Build history of the part. All positions in model axes, mm. Face numbers are marked on the shaded views. A direction names the side the tool comes from. Coordinates: 2 decimals unless noted, no trailing zeros. Write each loop counter-clockwise with the first axis right and the second up, starting at its lowest first coordinate (ties: lowest second). Pieces come first, ordered by that corner, then holes.
Autodesk Inventor part; units mm, degrees
ref_plane "YZ Plane" through (0, 0, 0) normal (1, 0, 0) x (0, 1, 0)
ref_plane "XZ Plane" through (0, 0, 0) normal (0, 1, 0) x (-1, 0, 0)
ref_plane "XY Plane" through (0, 0, 0) normal (0, 0, 1) x (1, 0, 0)
sketch "Sketch1" plane through (0, 0, 0) normal (0, 1, 0) x (-1, 0, 0)
  line L0 (10.6592, 57.15) -> (-7.8828, 57.15)
  line L1 (-7.8828, 57.15) -> (-7.8828, -12.7)
  line L2 (-7.8828, -12.7) -> (10.6592, -12.7)
  line L3 (10.6592, 50.8) -> (-1.5328, 50.8)
  line L4 (-1.5328, 50.8) -> (-1.5328, 25.4)
  line L5 (-1.5328, 25.4) -> (10.6592, 25.4)
  line L6 (10.6592, 19.05) -> (-1.5328, 19.05)
  line L7 (-1.5328, 19.05) -> (-1.5328, -6.35)
  line L8 (-1.5328, -6.35) -> (10.6592, -6.35)
  line L9 (10.6592, -12.7) -> (10.6592, -6.35)
  line L10 (10.6592, 19.05) -> (10.6592, 25.4)
  line L11 (10.6592, 50.8) -> (10.6592, 57.15)
  point P0 (0, 0)
  dimension "d0" = 18.542
  dimension "d3" = 6.35
  dimension "d4" = 6.35
  dimension "d5" = 6.35
  dimension "d7" = 0
  dimension "d8" = 25.4
  dimension "d9" = 25.4
  dimension "d25" = 0
  dimension "d26" = 0
extrude "Extrusion1" add sketch "Sketch1" along normal blind 101.6
sketch "Sketch2" plane through (1.5328, 0, -6.35) normal (-1, 0, 0) x (0, 0, 1)
  line L0 (0, 0) -> (0, 101.6)
  line L1 (0, 0) -> (25.4, 0)
  point P0 (6.35, 0)
  point P1 (12.7, 25.4)
  point P2 (12.7, 50.8)
  point P3 (12.7, 76.2)
  dimension "d12" = 12.7
  dimension "d13" = 25.4
  dimension "d14" = 25.4
  dimension "d15" = 0
  dimension "d16" = 0
  dimension "d17" = 25.4
hole "Hole1" at (1.5328, 25.4, 6.35) at (1.5328, 50.8, 6.35) at (1.5328, 76.2, 6.35) direction (1, 0, 0) diameter 4.826 depth 25.4 tip angle 118
sketch "Sketch3" plane through (0, 101.6, 0) normal (0, 1, 0) x (1, 0, 0)
  line L0 (1.5328, -25.4) -> (-10.7917, -24.9696)
  line L1 (-10.7917, -24.9696) -> (-10.7917, -25.4)
  line L2 (-10.6592, -25.4) -> (1.5328, -25.4)
  line L3 (-10.7917, -25.4) -> (1.5328, -25.4)
  point P0 (0, 0)
  dimension "d27" = 2
extrude "Extrusion2" cut sketch "Sketch3" against normal blind 111.125
sketch "Sketch4" plane through (0, 101.6, 0) normal (0, 1, 0) x (1, 0, 0)
  line L0 (1.5328, -50.8) -> (-12.9577, -50.8)
  line L1 (-12.9577, -50.8) -> (-12.9577, -51.306)
  line L2 (-12.9577, -51.306) -> (1.5328, -50.8)
  point P0 (0, 0)
  dimension "d30" = 2
extrude "Extrusion3" cut sketch "Sketch4" against normal blind 119.0625
sketch "Sketch5" plane through (0, 101.6, 0) normal (0, 1, 0) x (1, 0, 0)
  line L0 (-10.6592, -57.15) -> (7.8828, -57.15)
  line L1 (7.8828, -57.15) -> (-13.0423, -56.4193)
  line L2 (-13.0423, -56.4193) -> (-13.0009, -57.15)
  line L3 (-13.0009, -57.15) -> (7.8828, -57.15)
  point P0 (0, 0)
  dimension "d33" = 2
extrude "Extrusion4" cut sketch "Sketch5" against normal blind 196.85
sketch "Sketch6" plane through (0, 101.6, 0) normal (0, 1, 0) x (1, 0, 0)
  line L0 (7.8828, 12.7) -> (-10.6592, 12.7)
  line L1 (7.8828, 12.7) -> (-16.8119, 12.7)
  line L2 (-16.8119, 12.7) -> (-16.8119, 11.8376)
  line L3 (7.8828, -57.15) -> (7.8828, 12.7)
  line L4 (-16.8119, 11.8376) -> (7.8828, 12.7)
  point P0 (0, 0)
  dimension "d36" = 2
extrude "Extrusion5" cut sketch "Sketch6" against normal blind 334.9625
equation "\"d0\" = ElvDelWidth"
equation "\"d3\" = ElvDelFrontTabLength"
equation "\"d4\" = ElvDelMiddleTabLength"
equation "\"d5\" = ElvDelFrontTabLength"
equation "\"d8\" = ElvBeamWidth"
equation "\"d9\" = ElvBeamWidth"
equation "\"d10\" = ElvDelHeight"
equation "\"ElvBeamWidth\" = 25.4"
equation "\"ElvDelWidth\" = 18.542"
equation "\"ElvDelHeight\" = 101.6"
equation "\"ElvDelFrontTabLength\" = 6.35"
equation "\"ElvDelDepth\" = 6.35"
equation "\"d2\" = ElvDelDepth"
equation "\"ElvCrossBeamLength\" = 304.8"
equation "\"ElvFixedBeamLength\" = 990.6"
equation "\"ElvMiddleBeamLength\" = 990.6"
equation "\"ElvFrontBeamLength\" = 990.6"
equation "\"ElvEndEffectLength\" = 431.8"
equation "\"ElvWallWidth\" = 1.5875"
equation "\"ElvTopBeamLength\" = 457.2"
equation "\"ElvHoleFromFront\" = 25.4"
equation "\"ElvHoleFromMid\" = 38.1"
equation "\"ElvHoleFromFixed\" = 50.8"
equation "\"ElvHoleFromBottom\" = 38.1"
equation "\"ElvRivetPlateLength\" = 76.2"
equation "\"ElvDelMiddleTabLength\" = 6.35"
properties part number "ElvDel" material "Acetal Resin, White"
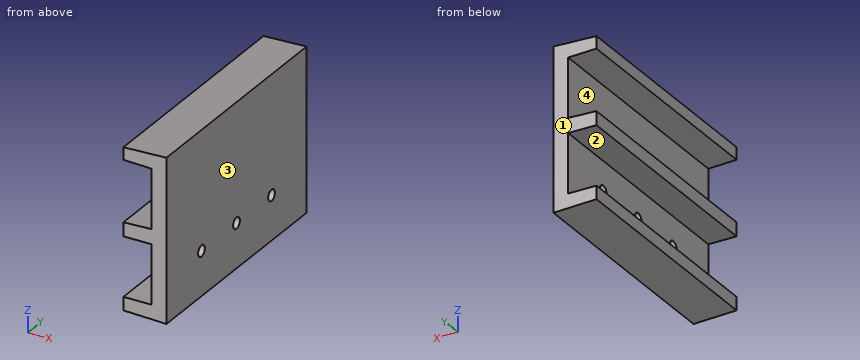
1. Probe line 1 along Z through (x, y) = (-10, 76); line 2 along Y through (x, z) = (5.75, 6.35); line 3 along Z through (x, y) = (-7, 66.5). List the from-to ranges inside material, lowest first.
Computed values:
line 1: z = -12.08 to -6.35, 19.05 to 25, 51.2 to 56.53
line 2: y = 0 to 22.99, 27.81 to 48.39, 53.21 to 73.79, 78.61 to 101.6
line 3: z = -12.18 to -6.35, 19.05 to 25.1, 51.1 to 56.63
2. Flat gauge pins, fed straight in: pin 1 (6 mm diameter, centred on x = -5, y = 38, fed in from -Z); pin 2 (1.5 mm diameter, centred on x = -4, y = 43.5, fed in from +Z); pin 3 (7.5 mm diameter, centred on y = 39.5, z = 6, fed in from -X). Where does each tip first touch, or does it go through?
Computed values:
pin 1: stops at z = -12.35
pin 2: stops at z = 56.76
pin 3: stops at x = 1.53
3. Saw through at C-C on x = -3.75. List the corners of the cut face in (y, z).
Computed values:
outline: (0, -12.29) - (101.6, -12.29) - (101.6, -6.35) - (0, -6.35) - close; (0, 19.05) - (101.6, 19.05) - (101.6, 25.22) - (0, 25.22) - close; (0, 50.98) - (101.6, 50.98) - (101.6, 56.74) - (0, 56.74) - close
4. Saw through at D-D on y = 41. List the corners of the cut face in (x, z).
Computed values:
outline: (-10.66, -12.05) - (7.88, -12.7) - (7.88, 57.15) - (-10.66, 56.5) - (-10.66, 51.23) - (1.53, 50.8) - (1.53, 25.4) - (-10.66, 24.97) - (-10.66, 19.05) - (1.53, 19.05) - (1.53, -6.35) - (-10.66, -6.35) - close
5. Saw through at A-A on z = 6.35. List the corners of the cut face in (x, y).
Computed values:
outline: (1.53, 0) - (7.88, 0) - (7.88, 22.99) - (1.53, 22.99) - close; (1.53, 27.81) - (7.88, 27.81) - (7.88, 48.39) - (1.53, 48.39) - close; (1.53, 53.21) - (7.88, 53.21) - (7.88, 73.79) - (1.53, 73.79) - close; (1.53, 78.61) - (7.88, 78.61) - (7.88, 101.6) - (1.53, 101.6) - close
6. Saw through at B-B on y = 25.4. List the corners of the cut face in (x, z).
Computed values:
outline: (-10.66, -12.05) - (7.88, -12.7) - (7.88, 3.94) - (1.53, 3.94) - (1.53, -6.35) - (-10.66, -6.35) - close; (-10.66, 19.05) - (1.53, 19.05) - (1.53, 8.76) - (7.88, 8.76) - (7.88, 57.15) - (-10.66, 56.5) - (-10.66, 51.23) - (1.53, 50.8) - (1.53, 25.4) - (-10.66, 24.97) - close
7. Mould opens along Z. For the marked faces 3 and 4 say: +Z half, -Z half, draft (parallel to the pull), parting line (faces both ways), or undercut.
Computed values:
face 3: draft
face 4: undercut
8. 3-axis set-ups, long thin cutter, end or side, ignore diameter. For the marked faces 1 and 2: which of +Z, -Z, +X, -X, +Y, -Y reach the whole face in a straight line?
Computed values:
face 1: +Z, -Z, +X, -X, +Y
face 2: -X, +Y, -Y
